Job drawing, mm, ordinate dimensions from the low corner. One solid piece. Coordinates: 2 decimals unless noted, no trailing zeros. Write each loop counter-clockwise with the first axis right and the second up, starting at its lowest first coordinate (ties: lowest second). Pieces come first, ordered by that corner, then holes. Notation, with made-up numbers: (35.25, -37.75) - (93.25, -37.75) arc R18 cw to (93.25, -25.75) - close; hole circle Ø10 at (-18.75, 26.25). An arc over 180 degrees is marked (long way). Use a Markdown table: item, result.
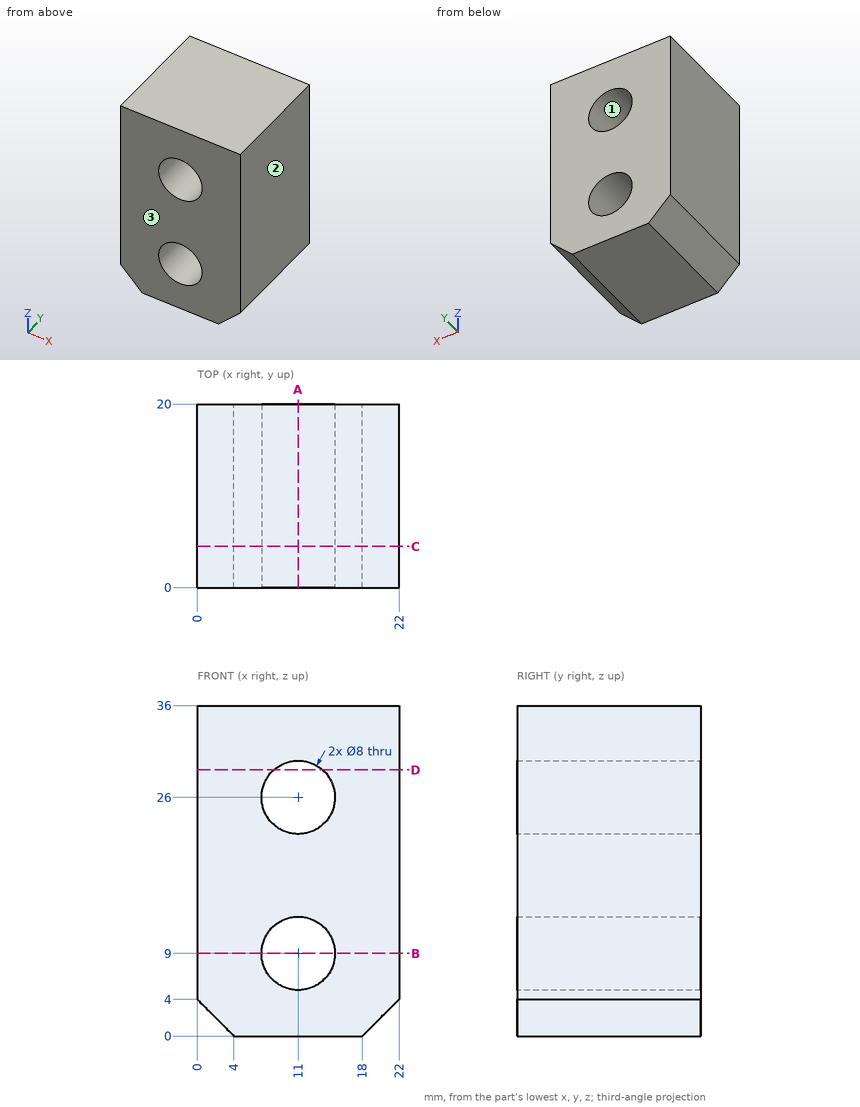
Item 1: Band-saw the part on B-B, the plane z = 9. Give the cut face in (x, y).
From the geometry:
| item | result |
|---|---|
| outline | (0, 0) - (7, 0) - (7, 20) - (0, 20) - close; (15, 0) - (22, 0) - (22, 20) - (15, 20) - close |
Item 2: Drop a flat-ended pin along its axis: P1, Ø1.5, axis at x = 6, y = 14, coming from the -Z side. Give the stop position or say it passes through.
From the geometry:
| item | result |
|---|---|
| P1 | z = 0 |
Item 3: Band-saw the part on D-D, the plane z = 29. Give the cut face in (x, y).
From the geometry:
| item | result |
|---|---|
| outline | (0, 0) - (8.35, 0) - (8.35, 20) - (0, 20) - close; (13.65, 0) - (22, 0) - (22, 20) - (13.65, 20) - close |
Item 4: Drill centre lines: probe 1 along X at (y, z) = (14, 9); probe 2 along Z at (x, y) = (7.5, 16.75); probe 3 along Z at (x, y) = (12, 5.5). Where is each one in solid material? Low to high.
From the geometry:
| item | result |
|---|---|
| probe 1 | 0 to 7, 15 to 22 |
| probe 2 | 0 to 7.06, 10.94 to 24.06, 27.94 to 36 |
| probe 3 | 0 to 5.13, 12.87 to 22.13, 29.87 to 36 |
Item 5: Band-saw the part on A-A, the plane x = 11. Give the cut face in (y, z).
From the geometry:
| item | result |
|---|---|
| outline | (0, 0) - (20, 0) - (20, 5) - (0, 5) - close; (0, 13) - (20, 13) - (20, 22) - (0, 22) - close; (0, 30) - (20, 30) - (20, 36) - (0, 36) - close |
Item 6: Two-plate mould, pull along X, no slides. Class the marked faces 1, 2 and 3: pulls with the +X half, pulls with the -X half, needs draft (parallel to the pull), parting line crosses it, or undercut.
From the geometry:
| item | result |
|---|---|
| face 1 | undercut |
| face 2 | pulls with the +X half |
| face 3 | needs draft |
Item 7: Band-saw the part on C-C, the plane y = 4.5. Give the cut face in (x, z), then the cut area to 3 significant figures.
From the geometry:
| item | result |
|---|---|
| outline | (0, 4) - (4, 0) - (18, 0) - (22, 4) - (22, 36) - (0, 36) - close; hole circle Ø8 at (11, 9); hole circle Ø8 at (11, 26) |
| area | 675 mm^2 |
